Model file for the job. Use its own axes, mm. Face numbers are marked on the shaded views. A direction names the side the tool comes from. Coordinates: 2 decimals unless noted, no trailing zeros. Order: outer loops, then holes, each group sorted by start corner. A loop starts at its lowest first (then second) coordinate and runs counter-clockwise, first axis right, second up.
from build123d import *

# Parameters (mm, degrees)
SKETCH1_R           = 55
BOSS_EXTRUDE1_DEPTH = 40
FILLET1_R           = 10
SKETCH2_R           = 12
CUT_EXTRUDE1_DEPTH  = 80
SKETCH3_R           = 82.5
CUT_EXTRUDE2_DEPTH  = 63
CHAMFER1_SIZE       = 2


with BuildPart() as part:
    # Sketch1 → Boss-Extrude1 (new, symmetric)
    with BuildSketch(Plane(origin=(0, 0, 0), x_dir=(1, 0, 0), z_dir=(0, 1, 0))):
        Polygon((-470, 0), (-445, 0), (445, 0), (470, 0), (470, 20), (445, 20), (445, 400), (345, 500), (-345, 500), (-445, 400), (-445, 20), (-470, 20), align=None)
        with Locations(Location((-316.5, 100, 0), (0, 0, 270))):
            Circle(SKETCH1_R, mode=Mode.SUBTRACT)
        with Locations(Location((316.5, 100, 0), (0, 0, 270))):
            Circle(SKETCH1_R, mode=Mode.SUBTRACT)
        with BuildLine():
            Line((-60, 225), (-60, 458))
            Line((-60, 458), (60, 458))
            Line((60, 458), (60, 225))
            ThreePointArc((60, 225), (0, 165), (-60, 225))
        make_face(mode=Mode.SUBTRACT)
    extrude(amount=BOSS_EXTRUDE1_DEPTH, both=True)

    # Fillet1
    fillet1_edges = [part.edges().sort_by_distance(p)[0] for p in [
        (445, 0, -20),
        (470, 0, -20),
        (-470, 0, -20),
        (-445, 0, -20),
    ]]
    fillet(fillet1_edges, radius=FILLET1_R)

    # Sketch2 → Cut-Extrude1 (cut)
    with BuildSketch(Plane.XY.offset(-458)):
        Circle(SKETCH2_R)
    extrude(amount=-CUT_EXTRUDE1_DEPTH, mode=Mode.SUBTRACT)

    # Sketch3 → Cut-Extrude2 (cut)
    with BuildSketch(Plane.XZ.offset(40)):
        with Locations(Location((-316.5, -100, 0), (0, 0, 270))):
            Circle(SKETCH3_R)
        with Locations(Location((316.5, -100, 0), (0, 0, 270))):
            Circle(SKETCH3_R)
    extrude(amount=-CUT_EXTRUDE2_DEPTH, mode=Mode.SUBTRACT)

    # Chamfer1
    chamfer1_edges = [part.edges().sort_by_distance(p)[0] for p in [
        (-316.5, 23, -17.5),
        (-316.5, -40, -17.5),
        (316.5, -40, -17.5),
        (316.5, 23, -17.5),
    ]]
    chamfer(chamfer1_edges, length=CHAMFER1_SIZE)


solid = part.part
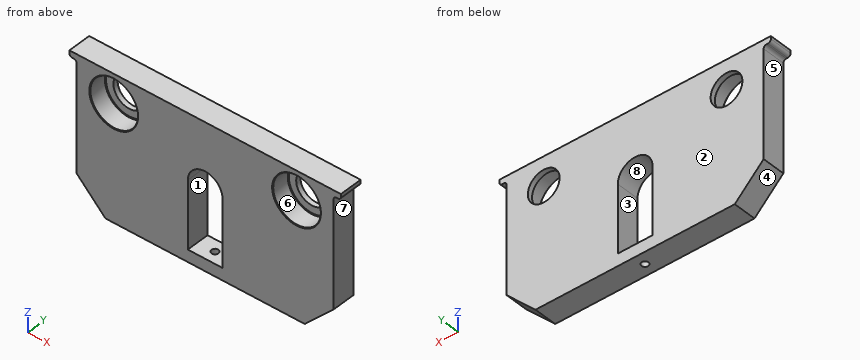
Q1. Drop flat-ended pins along their axis: P1, Ø6, axis at x = 27.5, y = 22, coming from the +Z side; P2, Ø6, axis at y = -21.5, z = -164, coming from the -X side; P3, Ø1.5, axis at x = 457.5, y = -4.5, coming from the -Z side; P4, Ø3, axis at y = 5.5, z = -209.5, coming from the +X side. Give the stop position or say it passes through.
Established:
P1: stops at z = 0
P2: stops at x = -445
P3: stops at z = -20
P4: stops at x = 445
Q2. Mould opens along Z. For the marked faces 1, 2, 3 and 4 say: pulls with the +Z half, pulls with the -Z half, needs draft (parallel to the pull), parting line crosses it, or undercut.
Established:
face 1: undercut
face 2: needs draft
face 3: undercut
face 4: pulls with the -Z half
Q3. Cut at D-D, the plane z = -269. List the corners of the cut face in (x, y).
Established:
outline: (-445, -40) - (-60, -40) - (-60, 40) - (-445, 40) - close; (60, -40) - (445, -40) - (445, 40) - (60, 40) - close
Q4. Cut at A-A, the plane z = -100. List the corners of the cut face in (x, y), plus the area to 3 significant figures.
Established:
outline: (-445, -40) - (-401, -40) - (-399, -38) - (-399, 21) - (-397, 23) - (-371.5, 23) - (-371.5, 40) - (-445, 40) - close; (-261.5, 23) - (-236, 23) - (-234, 21) - (-234, -38) - (-232, -40) - (232, -40) - (234, -38) - (234, 21) - (236, 23) - (261.5, 23) - (261.5, 40) - (-261.5, 40) - close; (371.5, 23) - (397, 23) - (399, 21) - (399, -38) - (401, -40) - (445, -40) - (445, 40) - (371.5, 40) - close
area: 46,700 mm2
Q5. Cut at C-C, the plane x = -316.5. List the corners of the cut face in (y, z).
Established:
outline: (-40, -500) - (40, -500) - (40, -155) - (23, -155) - (23, -180.5) - (21, -182.5) - (-38, -182.5) - (-40, -184.5) - close; (-40, -15.5) - (-38, -17.5) - (21, -17.5) - (23, -19.5) - (23, -45) - (40, -45) - (40, 0) - (-40, 0) - close
Q6. Cut at B-B, the plane y = 0. List the corners of the cut face in (x, z).
Established:
outline: (-470, -10) arc R10 ccw to (-460, -20) - (-455, -20) arc R10 cw to (-445, -30) - (-445, -400) - (-345, -500) - (-12, -500) - (-12, -458) - (-60, -458) - (-60, -225) arc R60 cw to (60, -225) - (60, -458) - (12, -458) - (12, -500) - (345, -500) - (445, -400) - (445, -30) arc R10 cw to (455, -20) - (460, -20) arc R10 ccw to (470, -10) - (470, 0) - (-470, 0) - close; hole circle Ø165 at (-316.5, -100); hole circle Ø165 at (316.5, -100)
Q7. Which spindle directions (+Z, -Z, +X, -X, +Y, -Y) get a long thin tool onto all of the face, cutting with end or side? Do the marked faces 5, 6, 7 and 8. Say none if no direction does.
Established:
face 5: -Z, -X, +Y, -Y
face 6: -Y
face 7: -Z, +X, +Y, -Y
face 8: +Y, -Y
Q8. Probe line 1 (X direction, y = 28.25, z = -100); line 2 (Z direction, x = 335, y = -15); line 3 (X direction, y = -23.5, z = -344). List the from-to ranges inside material, lowest first.
Established:
line 1: x = -445 to -371.5, -261.5 to 261.5, 371.5 to 445
line 2: z = -500 to -180.4, -19.6 to 0
line 3: x = -445 to -60, 60 to 445
